Read the model definition and answer for the solid it produces. Units are mm, in the model's axes. Coordinates: 2 decimals unless noted, no trailing zeros. Write each loop counter-clockwise with the first axis right and the second up, starting at its lowest first coordinate (ties: lowest second). Pieces come first, ordered by that corner, then holes. Notation, with made-up numbers: (-1.5, 61) -> (16.5, 61) arc R28 cw to (16.5, 93) -> close; hole circle Ø11 at (6.5, 78.25). An arc over 180 degrees is marked (long way). Answer in a Markdown table with one row per item. Add a question column.
Item 1: Straight lines are drawn through the part: line 1 (Z direction, x = -12.7, y = 0.8); line 2 (X direction, y = 1.05, z = 12.7); line 3 (Z direction, x = -63.5, y = 0.4). For each, find the intervals that lie inside material, in ascending order. Write a range as from..to.
Item 2: Section D-D on z = 88.9 is taken. Write down the section's boundary in (x, y).
Item 3: Section B-B on z = 12.7 is taken. Write down the section's boundary in (x, y).
Item 4: Section C-C on y = 1.2 is taken. Count the separate pieces of the cut face and the enclosed holes in it, then the cut area to 3 significant figures.
Item 5: Given pin 1 Ø5.5 at (x, z) = (-38.1, 12.7) entering from +Y; pin 2 Ø0.5 at (x, y) = (-70.5, 0.5) entering from +Z; pin 3 Ø0.8 at (y, z) = (0.5, 35.5) entering from -X; pin 4 Ø0.8 at (y, z) = (1, 64.5) entering from -X, each flat-ended and moving along its own axis, determine where each tip first touches the part or whether it passes through.
Item 6: Section A-A on x = -12.7 is taken. Write down the section's boundary in (y, z), then the cut area to 3 significant figures.
```python
from build123d import *

# Parameters (mm, degrees)
BOSS_EXTRUDE1_DEPTH = 1.5875
FILLET1_R           = 2.54
SKETCH2_R           = 2.4892
CUT_EXTRUDE1_DEPTH  = 2.5875
LPATTERN1_COUNT     = 3
LPATTERN1_PITCH     = 25.4
LPATTERN2_COUNT     = 3
LPATTERN2_PITCH     = 25.4


with BuildPart() as part:
    # Sketch1 → Boss-Extrude1 (new body)
    with BuildSketch(Plane(origin=(0, 0, 0), x_dir=(1, 0, 0), z_dir=(0, 1, 0))):
        Polygon((0, -26.9875), (-26.9875, -26.9875), (-26.9875, 0), (-101.6, 0), (-101.6, -26.9875), (-26.9875, -101.6), (0, -101.6), align=None)
        Polygon((-85.226987758, -25.4), (-25.4, -85.226987758), (-25.4, -44.45), (-44.45, -44.45), (-44.45, -25.4), align=None, mode=Mode.SUBTRACT)
    extrude(amount=BOSS_EXTRUDE1_DEPTH)

    # Fillet1
    fillet1_edges = [part.edges().sort_by_distance(p)[0] for p in [
        (-26.9875, 0.79375, 26.9875),
        (0, 0.79375, 26.9875),
        (0, 0.79375, 101.6),
        (-26.9875, 0.79375, 101.6),
        (-101.6, 0.79375, 26.9875),
        (-101.6, 0.79375, 0),
        (-26.9875, 0.79375, 0),
        (-44.45, 0.79375, 25.4),
        (-85.226987758, 0.79375, 25.4),
        (-25.4, 0.79375, 85.226987758),
        (-25.4, 0.79375, 44.45),
        (-44.45, 0.79375, 44.45),
    ]]
    fillet(fillet1_edges, radius=FILLET1_R)

    # Sketch2 → Cut-Extrude1 (cut, through all)
    with BuildSketch(Plane(origin=(0, 1.5875, 0), x_dir=(1, 0, 0), z_dir=(0, 1, 0))):
        with Locations((-88.9, -12.7)):
            Circle(SKETCH2_R)
        with Locations((-12.7, -88.9)):
            Circle(SKETCH2_R)
    cut_extrude1 = extrude(amount=-CUT_EXTRUDE1_DEPTH, mode=Mode.SUBTRACT)

    # LPattern1: Cut-Extrude1 ×3
    with Locations(*[(i * LPATTERN1_PITCH, 0, 0) for i in range(1, LPATTERN1_COUNT)]):
        add(cut_extrude1, mode=Mode.SUBTRACT)

    # LPattern2: Cut-Extrude1 ×3
    with Locations(*[(0, 0, -i * LPATTERN2_PITCH) for i in range(1, LPATTERN2_COUNT)]):
        add(cut_extrude1, mode=Mode.SUBTRACT)


solid = part.part
```
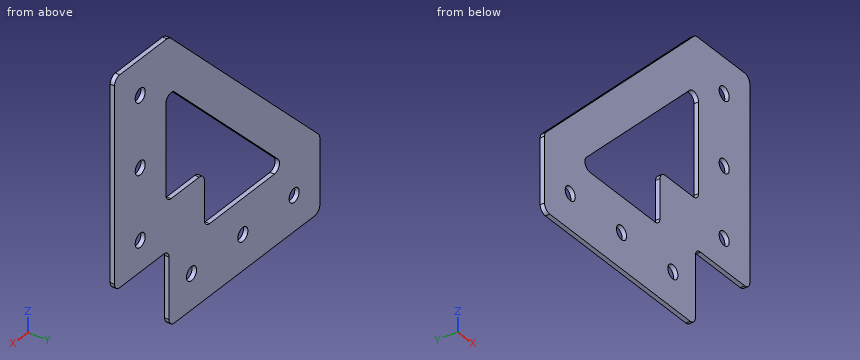
Results below:
| question | item | result |
|---|---|---|
| 1 | line 1 | z = 26.99..35.61, 40.59..61.01, 65.99..86.41, 91.39..101.6 |
| 1 | line 2 | x = -101.6..-91.39, -86.41..-65.99, -61.01..-40.59, -35.61..-26.99 |
| 1 | line 3 | z = 0..10.21, 15.19..25.4, 47.13..65.09 |
| 2 | outline | (-39.69, 0) -> (-15.19, 0) -> (-15.19, 1.59) -> (-39.69, 1.59) -> close; (-10.21, 0) -> (0, 0) -> (0, 1.59) -> (-10.21, 1.59) -> close |
| 3 | outline | (-101.6, 0) -> (-91.39, 0) -> (-91.39, 1.59) -> (-101.6, 1.59) -> close; (-86.41, 0) -> (-65.99, 0) -> (-65.99, 1.59) -> (-86.41, 1.59) -> close; (-61.01, 0) -> (-40.59, 0) -> (-40.59, 1.59) -> (-61.01, 1.59) -> close; (-35.61, 0) -> (-26.99, 0) -> (-26.99, 1.59) -> (-35.61, 1.59) -> close |
| 4 | separate pieces | 1 |
| 4 | enclosed holes | 7 |
| 4 | area | 5,280 mm2 |
| 5 | pin 1 | stops at y = 1.59 |
| 5 | pin 2 | stops at z = 58.34 |
| 5 | pin 3 | stops at x = -93.49 |
| 5 | pin 4 | stops at x = -64.49 |
| 6 | outline | (0, 26.99) -> (1.59, 26.99) -> (1.59, 35.61) -> (0, 35.61) -> close; (0, 40.59) -> (1.59, 40.59) -> (1.59, 61.01) -> (0, 61.01) -> close; (0, 65.99) -> (1.59, 65.99) -> (1.59, 86.41) -> (0, 86.41) -> close; (0, 91.39) -> (1.59, 91.39) -> (1.59, 101.6) -> (0, 101.6) -> close |
| 6 | area | 94.7 mm2 |
